Geometry check sheet. Reference: drawing and pictorial views, mm from the part's lowest x, y, z. A direction names the side the tool comes from. Give positions to 0.01 mm unless a question says otherwise; leave off trailing zeros. Order: outer loops, then holes, each group sorted by start corner. A loop starts at its lowest first (then second) coordinate and runs counter-clockwise, first axis right, second up. Notation, with made-up numbers: (35.5, 73.5) - (90.5, 73.5) arc R19 cw to (90.5, 81.5) - close; hole circle Ø4 at (10, -32.75). An arc over 180 degrees is marked (long way). Answer in a Markdown table with one row per item.
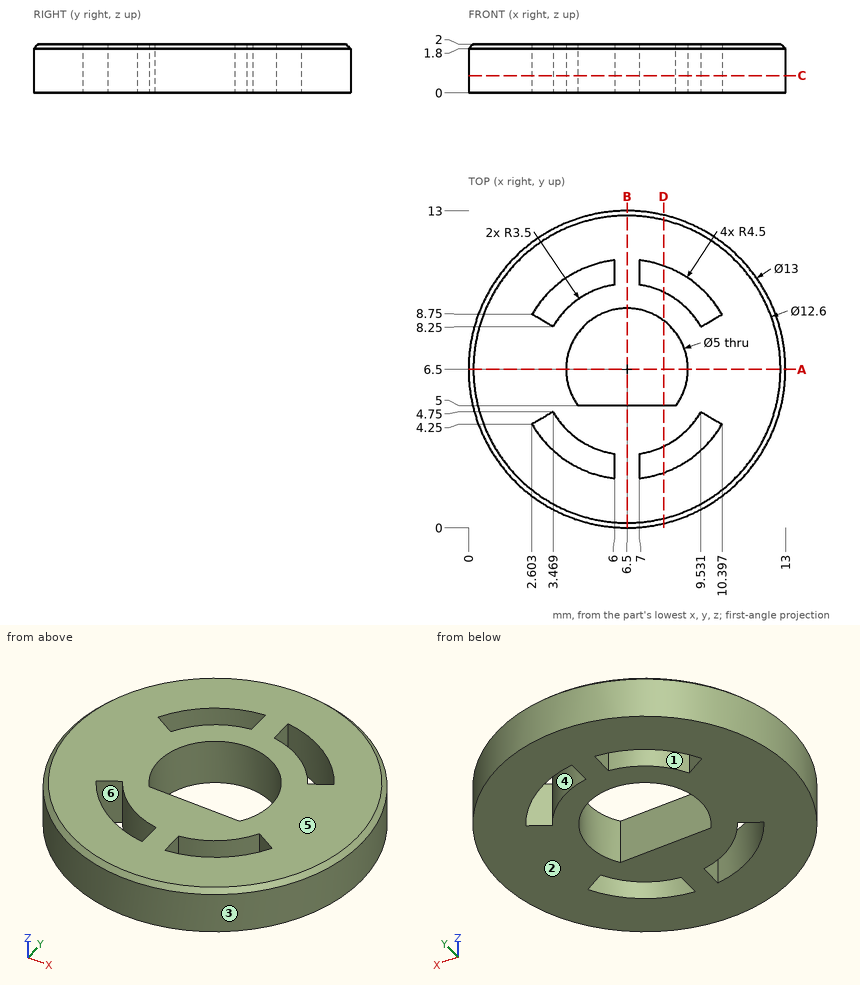
(1) Mould release check, pull along Y, two halves, no side actions. Record for the marked faces 1, 2, 3 and 4: pulls with the +Y half, pulls with the -Y half, needs draft (parallel to the pull), parting line crosses it, or undercut.
Geometry says:
| item | result |
|---|---|
| face 1 | undercut |
| face 2 | needs draft |
| face 3 | parting line crosses it |
| face 4 | undercut |
(2) Gauge pin test, flat ends, axial feed: P1, Ø0.5, axis at y = 2.5, z = 1, coming from the +X side; P2, Ø0.8, axis at y = 3, z = 1, coming from the -X side; P3, Ø0.8, axis at y = 10.5, z = 0.5, coming from the -X side. Record the tip position at first contact, or that the pin passes through.
Geometry says:
| item | result |
|---|---|
| P1 | x = 11.81 |
| P2 | x = 0.79 |
| P3 | x = 1.09 |
(3) Access from +Z, -Z, +X, -X, +Y, -Y to the whole of each face (thin tool, end or side, straight path). Record for the marked faces 5 and 6.
Geometry says:
| item | result |
|---|---|
| face 5 | +Z, +X, -X, +Y, -Y |
| face 6 | +Z, -Z |
(4) Cross-section at D-D, the plane x = 8. Give the number of separate pieces and of enclosed holes in the cut face, then the cut area to 3 significant figures.
Geometry says:
| item | result |
|---|---|
| separate pieces | 4 |
| enclosed holes | 0 |
| area | 13.9 mm² |
(5) Thickness scan on L1, parallel to X at y = 8.5, z = 1.95 (1 decimal); L2, parallel to X at y = 3, z = 1.15; L3, parallel to X at y = 2.5, z = 1.3. Record the ranges inside material, lowest first.
Geometry says:
| item | result |
|---|---|
| L1 | 0.5 to 3, 3.6 to 5, 8 to 9.4, 10 to 12.5 |
| L2 | 1.02 to 3.67, 6 to 7, 9.33 to 11.98 |
| L3 | 1.38 to 4.44, 6 to 7, 8.56 to 11.62 |
(6) Cross-section at A-A, the plane y = 6.5. Record the cut outline in (x, z), then the cut area to 3 significant figures.
Geometry says:
| item | result |
|---|---|
| outline | (0, 0) - (4, 0) - (4, 2) - (0.2, 2) - (0, 1.8) - close; (9, 0) - (13, 0) - (13, 1.8) - (12.8, 2) - (9, 2) - close |
| area | 16.0 mm² |
(7) Cross-section at C-C, the plane z = 0.7. Record the cut outline in (x, y).
Geometry says:
| item | result |
|---|---|
| outline | circle Ø13 at (6.5, 6.5); hole (2.6, 4.25) arc R4.5 ccw to (6, 2.03) - (6, 3.04) arc R3.5 cw to (3.47, 4.75) - close; hole (2.6, 8.75) - (3.47, 8.25) arc R3.5 cw to (6, 9.96) - (6, 10.97) arc R4.5 ccw to start; hole (4.5, 5) - (8.5, 5) arc R2.5 ccw (long way) to start; hole (7, 2.03) arc R4.5 ccw to (10.4, 4.25) - (9.53, 4.75) arc R3.5 cw to (7, 3.04) - close; hole (7, 9.96) arc R3.5 cw to (9.53, 8.25) - (10.4, 8.75) arc R4.5 ccw to (7, 10.97) - close |
(8) Cross-section at B-B, the plane x = 6.5. Record the cut outline in (y, z).
Geometry says:
| item | result |
|---|---|
| outline | (0, 0) - (5, 0) - (5, 2) - (0.2, 2) - (0, 1.8) - close; (9, 0) - (13, 0) - (13, 1.8) - (12.8, 2) - (9, 2) - close |
